For this review, take the finished solid that the model builds, in its own axes (mm). A direction names the side the tool comes from. Give positions to 0.01 mm unless a question says otherwise; leave off trailing zeros. Loops run counter-clockwise (first coordinate to the right, second up) from the corner with the lowest first, then second, coordinate; pieces in that order, holes last. Notation, with made-up numbers: (57.25, 72) - (107.25, 72) arc R25 cw to (107.25, 107) - close; hole circle Ø8 at (-12, 53.5). An arc over 180 degrees is marked (long way). Answer in a Markdown table with one row per item.
```python
from build123d import *

# Parameters (mm, degrees)
SKETCH1_R               = 350
SKETCH1_R_2             = 200
BOSS_EXTRUDE2_DEPTH     = 400
CUT_EXTRUDE2_DEPTH      = 637.396103068
CUT_EXTRUDE2_DEPTH_BACK = 637.396103068
SKETCH2_W               = 100
SKETCH2_H               = 40
CUT_EXTRUDE3_DEPTH      = 637.396103068
CUT_EXTRUDE3_DEPTH_BACK = 637.396103068
SKETCH3_W               = 40
SKETCH3_H               = 100
BOSS_EXTRUDE3_START     = 10
SKETCH6_R               = 350
BOSS_EXTRUDE3_DEPTH     = 10
SKETCH7_R               = 75
BOSS_EXTRUDE4_DEPTH     = 150
SKETCH9_R               = 250
BOSS_EXTRUDE5_DEPTH     = 150
FILLET1_R               = 250
FILLET3_R               = 250
FILLET4_R               = 250


with BuildPart() as part:
    # Sketch1 → Boss-Extrude2 (new body)
    with BuildSketch(Plane.XY):
        Circle(SKETCH1_R)
        Circle(SKETCH1_R_2, mode=Mode.SUBTRACT)
    extrude(amount=BOSS_EXTRUDE2_DEPTH)

    # Sketch2 → Cut-Extrude2 (cut, two sides: drawn at the far end of the back side and taken through both)
    with BuildSketch(Plane(origin=(0, 0, 0), x_dir=(1, 0, 0), z_dir=(0, 1, 0)).offset(-CUT_EXTRUDE2_DEPTH_BACK)):
        with Locations((0, -200)):
            Rectangle(SKETCH2_W, SKETCH2_H)
    extrude(amount=CUT_EXTRUDE2_DEPTH + CUT_EXTRUDE2_DEPTH_BACK, mode=Mode.SUBTRACT)

    # Sketch3 → Cut-Extrude3 (cut, two sides: drawn at the far end of the back side and taken through both)
    with BuildSketch(Plane(origin=(0, 0, 0), x_dir=(0, 0, -1), z_dir=(1, 0, 0)).offset(-CUT_EXTRUDE3_DEPTH_BACK)):
        with Locations((-200, 0)):
            Rectangle(SKETCH3_W, SKETCH3_H)
    extrude(amount=CUT_EXTRUDE3_DEPTH + CUT_EXTRUDE3_DEPTH_BACK, mode=Mode.SUBTRACT)

    # Sketch6 → Boss-Extrude3 (add)
    with BuildSketch(Plane(origin=(0, 0, 0), x_dir=(-1, 0, 0), z_dir=(0, 0, -1)).offset(BOSS_EXTRUDE3_START)):
        Circle(SKETCH6_R)
    extrude(amount=-BOSS_EXTRUDE3_DEPTH)

    # Loft4: read off the stored shape, not the designer's step
    # Loft4: loft between two sections, ruled curve by curve
    loft4_from = [
        Edge.make_bspline([(170.39658005, -104.713922223, -150), (379.824424496, 236.079237876, -150), (39.031264397, 445.507082323, -150), (-170.39658005, 104.713922223, -150), (-379.824424496, -236.079237876, -150), (-39.031264397, -445.507082323, -150), (170.39658005, -104.713922223, -150)], [0, 0, 0, 0, 0.5, 0.5, 0.5, 1, 1, 1, 1], 3, [1, 0.333333333, 0.333333333, 1, 0.333333333, 0.333333333, 1]),
    ]
    loft4_to = [
        Edge.make_bspline([(327.249685966, -124.127527305, -10), (575.504740577, 530.371844627, -10), (-78.994631356, 778.626899238, -10), (-327.249685966, 124.127527305, -10), (-575.504740577, -530.371844627, -10), (78.994631356, -778.626899238, -10), (327.249685966, -124.127527305, -10)], [0, 0, 0, 0, 0.5, 0.5, 0.5, 1, 1, 1, 1], 3, [1, 0.333333333, 0.333333333, 1, 0.333333333, 0.333333333, 1]),
    ]
    loft4 = Solid(Shell([*[Face.make_surface_from_curves(loft4_from[k], loft4_to[k]) for k in range(1)], Face(Wire(loft4_from)), Face(Wire(loft4_to))]))
    add(loft4)

    # Sketch7 → Boss-Extrude4 (add)
    with BuildSketch(Plane(origin=(0, 0, -150), x_dir=(-1, 0, 0), z_dir=(0, 0, -1))):
        Circle(SKETCH7_R)
    extrude(amount=BOSS_EXTRUDE4_DEPTH)

    # Sketch9 → Boss-Extrude5 (add)
    with BuildSketch(Plane(origin=(0, 0, -300), x_dir=(-1, 0, 0), z_dir=(0, 0, -1))):
        Circle(SKETCH9_R)
    extrude(amount=BOSS_EXTRUDE5_DEPTH)

    # Fillet1
    # the kernel refuses this fillet: 250 mm, written as the material it takes off along each edge
    with BuildSketch(Plane(origin=(0, 0, -450), x_dir=(-1, 0, 0), z_dir=(0, -1, 0))) as fillet1_piece_1:
        with BuildLine():
            CenterArc((20.871215252, -250), FILLET1_R, 23.578178478, 66.421821522)
            Line((20.871215252, 0), (20.871215252, 5))
            Line((20.871215252, 5), (250, 5))
            Line((250, 5), (255, 0))
            ThreePointArc((255, 0), (255, -75), (254.582575695, -148))
            Line((254.582575695, -148), (250, -150))
        make_face()
    revolve(axis=Axis((0, 0, -450), (0, 0, -1)), mode=Mode.SUBTRACT)

    # Fillet3
    # the kernel refuses this fillet: 250 mm, written as the material it takes off along each edge
    with BuildSketch(Plane(origin=(0, 0, -150), x_dir=(0.8519829002496553, -0.5235696111141154, 0), z_dir=(-0.5235696111141154, -0.8519829002496553, 0))) as fillet3_piece_1:
        with BuildLine():
            CenterArc((100.318750936, 250), FILLET3_R, 270, 42.94225565)
            Line((270.633984519, 66.989833043), (274.04028919, 63.329629703))
            ThreePointArc((274.04028919, 63.329629703), (238.570984694, 30.057815333), (203.487874785, -3.582559069))
            Line((203.487874785, -3.582559069), (200, -5))
            Line((200, -5), (100.318750936, -5))
            Line((100.318750936, -5), (100.318750936, 0))
        make_face()
    revolve(axis=Axis((0, 0, -150), (0, 0, 1)), mode=Mode.SUBTRACT)

    # Fillet4
    # the kernel refuses this fillet: 250 mm, written as the material it takes off along each edge
    with BuildSketch(Plane(origin=(0, 0, -10), x_dir=(-1, 0, 0), z_dir=(0, -1, 0))) as fillet4_piece_1:
        with BuildLine():
            CenterArc((100, -109.702841138), FILLET4_R, 0, 46.957870566)
            Line((350, -109.702841138), (355, -109.702841138))
            Line((355, -109.702841138), (355, 0))
            Line((355, 0), (353.36883922, 3.694715457))
            ThreePointArc((353.36883922, 3.694715457), (313.60959417, 40.086717001), (274.046664209, 76.664427119))
            Line((274.046664209, 76.664427119), (270.633984518, 73.010166957))
        make_face()
    revolve(axis=Axis((0, 0, -10), (0, 0, -1)), revolution_arc=200.772, mode=Mode.SUBTRACT)
    with BuildSketch(Plane(origin=(0, 0, -10), x_dir=(0.9349991027611482, -0.35465007801472115, 0), z_dir=(0.35465007801472115, 0.9349991027611482, 0))) as fillet4_piece_2:
        with BuildLine():
            CenterArc((100, -109.702841138), FILLET4_R, 0, 46.957870566)
            Line((350, -109.702841138), (355, -109.702841138))
            Line((355, -109.702841138), (355, 0))
            Line((355, 0), (353.36883922, 3.694715457))
            ThreePointArc((353.36883922, 3.694715457), (313.60959417, 40.086717001), (274.046664209, 76.664427119))
            Line((274.046664209, 76.664427119), (270.633984519, 73.010166957))
        make_face()
    revolve(axis=Axis((0, 0, -10), (0, 0, -1)), revolution_arc=159.228, mode=Mode.SUBTRACT)


solid = part.part
```
1. For faces 1 (the face through (-1, 271, 220)), 2 (the face through (0, 0, -450)), 3 (the face through (-271, -50, 200)), 4 (the face through (3, 3, 0)), 5 (the face through (14, -74, -150)), list the 3-axis set-ups (+Z, -Z, +X, -X, +Y, -Y) from which the entire face can be reached by the end or side of a thin tool; tool diameter is ignored.
Values:
| item | result |
|---|---|
| face 1 | +Y, -Y |
| face 2 | -Z, +X, -X, +Y, -Y |
| face 3 | +X, -X |
| face 4 | +Z |
| face 5 | none |
2. Wall thickness on line 1 (Y direction, x = 0, z = 287); line 2 (Z direction, x = -222.5, y = 65): over which ranges is each line inside the solid? List them lowest first. Write a range as [from, to].
Values:
| item | result |
|---|---|
| line 1 | y = [-350, -200], [200, 350] |
| line 2 | z = [-334.2, -300], [-112.63, 400] |
3. Mouldability with a two-part tool opening along X and no side actions: class faces 6 (the face through (151, -151, 400)), 7 (the face through (190.764, 60.075, 197.2)) as released by +X, released by -X, zero draft, split by the parting line, or undercut.
Values:
| item | result |
|---|---|
| face 6 | zero draft |
| face 7 | undercut |
4. We need section B-B, the plane x = 0. Count the separate pieces of the cut face and the enclosed holes in it, and give its area (3 significant figures).
Values:
| item | result |
|---|---|
| separate pieces | 3 |
| enclosed holes | 0 |
| area | 265,000 mm^2 |
5. Clearance check with flat-ended pins moving along their axes: pin 1 (10 mm diameter, centred on x = -136, y = 134, fed in from +Z); pin 2 (12 mm diameter, centred on x = 302.5, z = 204.5, fed in from -Y); pin 3 (1 mm diameter, centred on y = -92, z = -119, fed in from +X). State where each tip first meets the part, or that it passes through.
Values:
| item | result |
|---|---|
| pin 1 | stops at z = 0 |
| pin 2 | stops at y = -185.98 |
| pin 3 | stops at x = 201.85 |
6. We need section A-A, the plane z = 114. Give the boundary of the cut face in (x, y), and give its area (3 significant figures).
Values:
| item | result |
|---|---|
| outline | circle Ø700 at (0, 0); hole circle Ø400 at (0, 0) |
| area | 259,000 mm^2 |
